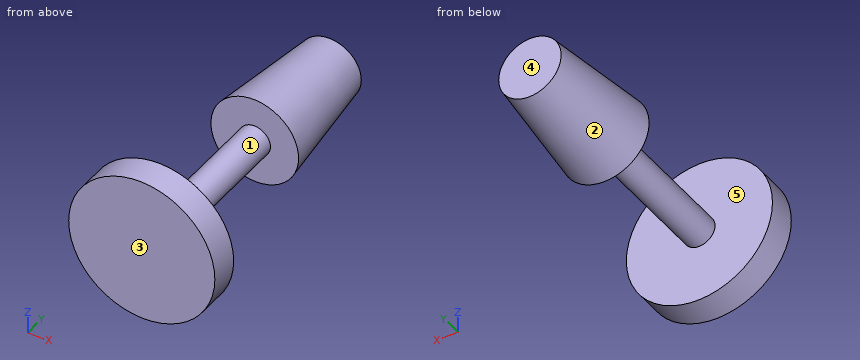
```python
from build123d import *

# Parameters (mm, degrees)
SKETCH3_W = 5
SKETCH3_H = 2


with BuildPart() as part:
    # Sketch1 → Revolve2 (revolve)
    with BuildSketch(Plane.XY):
        Polygon((0, -8.647232081), (0, 11.352767919), (2.135, 11.352767919), (3, 3.352767919), (1.071676077, 3.352767919), (1.071676077, -8.647232081), align=None)
    revolve(axis=Axis((0, -8.647232081, 0), (0, 1, 0)))

    # Sketch3 → Revolve3 (revolve)
    with BuildSketch(Plane.XY):
        with Locations((2.5, -7.647232081)):
            Rectangle(SKETCH3_W, SKETCH3_H)
    revolve(axis=Axis((0, -8.647232081, 0), (0, 1, 0)))


solid = part.part
```
The listing builds one solid part. Answer for the finished solid, in the listing's coordinates (mm). Face numbers are marked on the shaded views. A direction names the side the tool comes from. Round coordinates to 2 decimals unless told otherwise and drop trailing zeros. Write each loop counter-clockwise with the first axis right and the second up, starting at its lowest first coordinate (ties: lowest second). Pieces come first, ordered by that corner, then holes. Notation, with made-up numbers: (-30.5, -19.75) -> (-3.5, -19.75) arc R24 ccw to (-3.5, 7.25) -> close; hole circle Ø11 at (40.5, 38). An arc over 180 degrees is marked (long way). Use CSV: the item, a comma, the result in double quotes. Start each with the question number.
(1) Which of the six approach directions +Z, -Z, +X, -X, +Y, -Y give full straight-line access (tool end or side, diameter ignored) to the marked faces 1 and 2?
(2) Section B-B on z = 0 is taken. Give the vertices of the cut face in (x, y) (3 decimals).
(3) The mould has two halves that part along Y. Classify the marked faces 3, 4 and 5: released by +Y, released by -Y, zero draft, split by the parting line, or undercut.
(4) Section D-D on x = -4 is taken. Give the vertices of the cut face in (y, z).
(5) Section C-C on y = -4.25 is taken. Give the vertices of the cut face in (x, z).
(6) Consider L1, parallel to Y at x = 0.5, z = -1; L2, parallel to X at y = 9.25, z = 1; L3, parallel to Y at x = 3.25, z = -3.5. Determine where each line is inside the solid, lowest interval first. Write a range as from..to.
(7) Section A-A on x = 0 is taken. Give the vertices of the cut face in (y, z) (3 decimals), then the cut area to 3 significant figures.
A:
1,face 1,"none"
1,face 2,"+Y"
2,outline,"(-5, -8.647) -> (5, -8.647) -> (5, -6.647) -> (1.072, -6.647) -> (1.072, 3.353) -> (3, 3.353) -> (2.135, 11.353) -> (-2.135, 11.353) -> (-3, 3.353) -> (-1.072, 3.353) -> (-1.072, -6.647) -> (-5, -6.647) -> close"
3,face 3,"released by -Y"
3,face 4,"released by +Y"
3,face 5,"undercut"
4,outline,"(-8.65, -3) -> (-6.65, -3) -> (-6.65, 3) -> (-8.65, 3) -> close"
5,outline,"circle Ø2.14 at (0, 0)"
6,L1,"y = -8.65..-6.65, 3.35..11.35"
6,L2,"x = -2.14..2.14"
6,L3,"y = -8.65..-6.65"
7,outline,"(-8.647, -5) -> (-6.647, -5) -> (-6.647, -1.072) -> (3.353, -1.072) -> (3.353, -3) -> (11.353, -2.135) -> (11.353, 2.135) -> (3.353, 3) -> (3.353, 1.072) -> (-6.647, 1.072) -> (-6.647, 5) -> (-8.647, 5) -> close"
7,area,"82.5 mm²"
